from build123d import *

# Parameters (mm, degrees)
F0_R     = 9.55
F0_W     = 12.8
F0_H     = 12.8
F1_DEPTH = 8.03


with BuildPart() as f1:
    # F0 (on Front) → F1 (new body)
    with BuildSketch(Plane.XZ):
        Circle(F0_R)
        Rectangle(F0_W, F0_H, mode=Mode.SUBTRACT)
    extrude(amount=F1_DEPTH)


solid = f1.part
Geometry check sheet. Reference: the model listing, model coordinates, mm. A direction names the side the tool comes from. Give positions to 0.01 mm unless a question says otherwise; leave off trailing zeros. Loops run counter-clockwise (first coordinate to the right, second up) from the corner with the lowest first, then second, coordinate; pieces in that order, holes last.
(1) Section check D-D on z = -6.75. Record the cut outline in (x, y).
From the geometry:
outline: (-6.76, -8.03) - (6.76, -8.03) - (6.76, 0) - (-6.76, 0) - close
(2) Thickness scan on L1, parallel to Z at x = -4, y = -3; L2, parallel to Z at x = -1.5, y = -2.5; L3, parallel to X at y = -7.25, z = 5. Record the ranges inside material, lowest first.
From the geometry:
L1: z = -8.67 to -6.4, 6.4 to 8.67
L2: z = -9.43 to -6.4, 6.4 to 9.43
L3: x = -8.14 to -6.4, 6.4 to 8.14
(3) Depth check by flat-ended pin: pin 1 Ø1.5 at (y, z) = (-3, -1.5) entering from -X; pin 2 Ø4 at (x, z) = (5.5, -5.5) entering from +Y; pin 3 Ø2 at (x, y) = (6.5, -6) entering from -Z; pin 4 Ø1 at (y, z) = (-5, 2.5) entering from -X. Enter the tip coordinate at first touch or a pass-through.
From the geometry:
pin 1: stops at x = -9.52
pin 2: stops at y = 0
pin 3: stops at z = -7.81
pin 4: stops at x = -9.34
(4) Set-up check for faces 1 (the flat face through (-7, -8.03, 1)), 2 (the flat face through (0, -4, 6.4)): record each of +Z, -Z, +X, -X, +Y, -Y from which the full face is reachable in a straight line by a thin tool's end or side.
From the geometry:
face 1: +Z, -Z, +X, -X, -Y
face 2: +Y, -Y
(5) Section check B-B on z = 0. Record the cut outline in (x, y).
From the geometry:
outline: (-9.55, -8.03) - (-6.4, -8.03) - (-6.4, 0) - (-9.55, 0) - close; (6.4, -8.03) - (9.55, -8.03) - (9.55, 0) - (6.4, 0) - close
(6) Section check A-A on x = 0. Record the cut outline in (y, z), then the cut area to 3 significant figures.
From the geometry:
outline: (-8.03, -9.55) - (0, -9.55) - (0, -6.4) - (-8.03, -6.4) - close; (-8.03, 6.4) - (0, 6.4) - (0, 9.55) - (-8.03, 9.55) - close
area: 50.6 mm2
(7) Section check C-C on y = -4. Record the cut outline in (x, z), then the cut area to 3 significant figures.
From the geometry:
outline: circle Ø19.1 at (0, 0); hole (-6.4, -6.4) - (6.4, -6.4) - (6.4, 6.4) - (-6.4, 6.4) - close
area: 123 mm2
(8) Release check for a two-part mould opening along X. For faces 3 (the flat face through (6.4, -4, 0)), 4 (the cylindrical face through (-7.58, -3.96, -5.81)), 5 (the flat face through (-7, 0, 1)) record: released by +X, released by -X, zero draft, split by the parting line, or undercut.
From the geometry:
face 3: undercut
face 4: split by the parting line
face 5: zero draft
